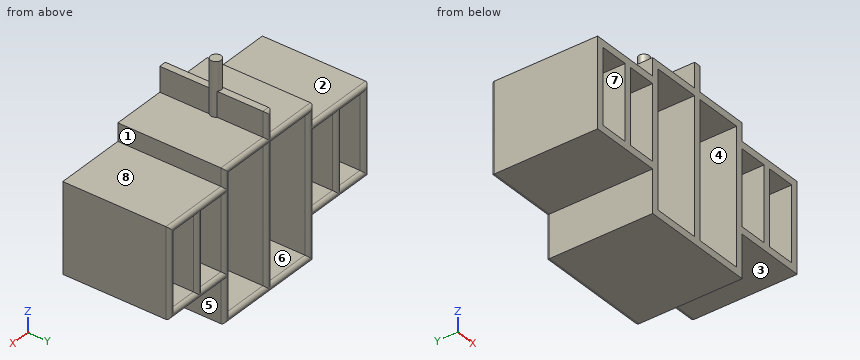
Autodesk Inventor part; units mm, degrees
ref_plane "YZ Plane" through (0, 0, 0) normal (1, 0, 0) x (0, 1, 0)
ref_plane "XZ Plane" through (0, 0, 0) normal (0, 1, 0) x (-1, 0, 0)
ref_plane "XY Plane" through (0, 0, 0) normal (0, 0, 1) x (1, 0, 0)
sketch "Szkic1" plane through (0, 0, 0) normal (0, 1, 0) x (-1, 0, 0)
  line L0 (16.25, 0) -> (-16.25, 0)
  line L1 (-16.25, 0) -> (-16.25, 2)
  line L2 (-16.25, 2) -> (16.25, 2)
  line L3 (16.25, 2) -> (16.25, 0)
  line L4 (-1, 2) -> (1, 2)
  line L5 (1, 2) -> (1, 49)
  line L6 (1, 49) -> (-1, 49)
  line L7 (-1, 49) -> (-1, 2)
  line L8 (16.25, 2) -> (14.25, 2)
  line L9 (14.25, 2) -> (14.25, 42)
  line L10 (14.25, 42) -> (16.25, 42)
  line L11 (16.25, 42) -> (16.25, 2)
  line L12 (-16.25, 2) -> (-14.25, 2)
  line L13 (-14.25, 2) -> (-14.25, 42)
  line L14 (-14.25, 42) -> (-16.25, 42)
  line L15 (-16.25, 42) -> (-16.25, 2)
  line L16 (14.25, 42) -> (1, 42)
  line L17 (1, 42) -> (1, 40)
  line L18 (1, 40) -> (14.25, 40)
  line L19 (14.25, 40) -> (14.25, 42)
  line L20 (-14.25, 42) -> (-1, 42)
  line L21 (-1, 42) -> (-1, 40)
  line L22 (-1, 40) -> (-14.25, 40)
  line L23 (-14.25, 40) -> (-14.25, 42)
  line L24 (16.25, 37) -> (36.25, 37)
  line L25 (36.25, 37) -> (36.25, 12)
  line L26 (36.25, 12) -> (16.25, 12)
  line L27 (16.25, 12) -> (16.25, 37)
  line L28 (-16.25, 37) -> (-36.25, 37)
  line L29 (-36.25, 37) -> (-36.25, 12)
  line L30 (-36.25, 12) -> (-16.25, 12)
  line L31 (-16.25, 12) -> (-16.25, 37)
  circle A0 centre (0, -31.074) radius 80.074
  line L32 (36.25, 37) -> (34.25, 37)
  line L33 (34.25, 37) -> (34.25, 12)
  line L34 (34.25, 12) -> (36.25, 12)
  line L35 (36.25, 12) -> (36.25, 37)
  line L36 (34.25, 37) -> (16.25, 37)
  line L37 (16.25, 37) -> (16.25, 35)
  line L38 (16.25, 35) -> (34.25, 35)
  line L39 (34.25, 35) -> (34.25, 37)
  line L40 (34.25, 12) -> (16.25, 12)
  line L41 (16.25, 12) -> (16.25, 14)
  line L42 (16.25, 14) -> (34.25, 14)
  line L43 (34.25, 14) -> (34.25, 12)
  line L44 (-16.25, 37) -> (-36.25, 37)
  line L45 (-36.25, 37) -> (-36.25, 35)
  line L46 (-36.25, 35) -> (-16.25, 35)
  line L47 (-16.25, 35) -> (-16.25, 37)
  line L48 (-16.25, 12) -> (-36.25, 12)
  line L49 (-36.25, 12) -> (-36.25, 14)
  line L50 (-36.25, 14) -> (-16.25, 14)
  line L51 (-16.25, 14) -> (-16.25, 12)
  line L52 (-36.25, 35) -> (-34.25, 35)
  line L53 (-34.25, 35) -> (-34.25, 14)
  line L54 (-34.25, 14) -> (-36.25, 14)
  line L55 (-36.25, 14) -> (-36.25, 35)
  line L56 (26.25, 35) -> (24.25, 35)
  line L57 (24.25, 35) -> (24.25, 14)
  line L58 (24.25, 14) -> (26.25, 14)
  line L59 (26.25, 14) -> (26.25, 35)
  line L60 (-24.25, 35) -> (-26.25, 35)
  line L61 (-26.25, 35) -> (-26.25, 14)
  line L62 (-26.25, 14) -> (-24.25, 14)
  line L63 (-24.25, 14) -> (-24.25, 35)
  point P0 (0, 0)
  point P1 (0, 0)
  point P2 (0, 2)
  point P3 (7.625, 40)
  point P4 (7.625, 42)
  point P5 (0, 49)
  point P6 (26.25, 37)
  point P7 (26.25, 14)
  point P8 (1, 42)
  point P9 (1, 48.9938)
  point P10 (-1, 48.9938)
  point P11 (-1, 42)
  point P12 (-16.25, 12)
  point P13 (16.25, 12)
  point P14 (-16.25, 14)
  point P15 (16.25, 14)
  dimension "d0" = 32.5
  dimension "d1" = 2
  dimension "d2" = 2
  dimension "d3" = 49
  dimension "d4" = 40
  dimension "d5" = 2
  dimension "d6" = 2
  dimension "d7" = 2
  dimension "d8" = 20
  dimension "d9" = 20
  dimension "d10" = 25
  dimension "d11" = 25
  dimension "d12" = 160.148
  dimension "d13" = 80.074
  dimension "d14" = 5
  dimension "d15" = 5
  dimension "d16" = 2
  dimension "d17" = 2
  dimension "d18" = 2
  dimension "d19" = 2
  dimension "d20" = 2
  dimension "d21" = 2
  dimension "d22" = 2
  dimension "d23" = 8
  dimension "d24" = 8
extrude "Wyciągnięcie proste1" add sketch "Szkic1" along normal blind 30 contours L0 L1 L2 L3 | L2 L9 L10 L11 | L15 L14 L13 L2 | L11 L42 L33 L26 | L30 L29 L50 L15 | L2 L7 A0 L5 | L18 L5 L16 L9 | L33 L24 L25 L26 | L13 L20 L7 L22 | L11 L24 L33 L38 | L57 L38 L59 L42 | L46 L29 L28 L15 | L50 L61 L46 L63 | L29 L46 L53 L50
sketch "Szkic2" plane through (1, 0, 42) normal (0, 0, 1) x (1, 0, 0)
  circle A0 centre (-1, 15) radius 1.5
  line L0 (0, 30) -> (15.25, 30)
  line L1 (0, 0) -> (0, 30)
  point P0 (-1, 0)
  dimension "d27" = 3
  dimension "d30" = 15
  dimension "d31" = 1
extrude "Wyciągnięcie proste2" add sketch "Szkic2" along normal blind 15
fillet "Zaokrąglenie1" radius 1 40 edges at (36.25, 30, 24.5) (34.25, 30, 24.5) (26.25, 30, 37) (30.25, 30, 35) (26.25, 30, 24.5) (20.25, 30, 35) (24.25, 30, 24.5) (30.25, 30, 14) (26.25, 30, 12) (20.25, 30, 14) (1, 30, 45.4969) (0, 30, 49) (-1, 30, 45.4969) (8.625, 30, 42) (16.25, 30, 39.5) (16.25, 30, 24.5) (14.25, 30, 21) (16.25, 30, 6) (7.625, 30, 2) (0, 30, 0) (1, 30, 21) (-1, 30, 21) (7.625, 30, 40) (-7.625, 30, 40) (-8.625, 30, 42) (-16.25, 30, 39.5) (-14.25, 30, 21) (-16.25, 30, 24.5) (-26.25, 30, 37) (-20.25, 30, 35) (-24.25, 30, 24.5) (-26.25, 30, 24.5) (-30.25, 30, 35) (-34.25, 30, 24.5) (-36.25, 30, 24.5) (-30.25, 30, 14) (-26.25, 30, 12) (-20.25, 30, 14) (-16.25, 30, 6) (-7.625, 30, 2)
equation "\"d5\" = d2"
equation "\"d6\" = d2"
equation "\"d9\" = d8"
equation "\"d11\" = d10"
equation "\"d15\" = d14"
equation "\"d16\" = d6"
equation "\"d19\" = d18"
equation "\"d22\" = d21"
properties part number "klapy"
Work out the finished part from the listing and answer in its coordinate system (mm). Face numbers are marked on the shaded views. A direction names the side the tool comes from. Coordinates: 2 decimals unless noted, no trailing zeros.
1) Consider probe 1 along X at (y, z) = (10, 9); probe 2 along Z at (x, y) = (-9.5, 16); probe 3 along X at (y, z) = (15, 36.5). Determine where each line is inside the solid, lowest interval first.
Results:
probe 1: x = -16.25 to -14.25, -1 to 1, 14.25 to 16.25
probe 2: z = 0 to 2, 40 to 42
probe 3: x = -36.25 to -14.25, -1 to 1, 14.25 to 36.25
2) For a pull along Z with two mould halves and no side action, classify the marked faces 5, 6, 7 and 8 as +Z half, -Z half, draft (parallel to the pull), parting line (faces both ways), or undercut.
Results:
face 5: draft
face 6: undercut
face 7: undercut
face 8: +Z half
3) For the marked faces 1, 2, 3 and 4, determine the directions among +Z, -Z, +X, -X, +Y, -Y from which every point of the face is accessible in a straight line to the end or side of a thin tool.
Results:
face 1: +Z, +X, +Y, -Y
face 2: +Z, -X, +Y, -Y
face 3: -Z, +X, +Y, -Y
face 4: +Y, -Y
4) Section B-B (z = 15.5) is taken. Give the number of separate pieces and of enclosed holes in the cut face, plus the area to 3 significant figures.
Results:
separate pieces: 7
enclosed holes: 0
area: 417 mm2
5) Flat-ended cylindrical pins translate along their axes: pin 1 (4.5 mm diameter, centred on x = -8, y = 13, fed in from +Z); pin 2 (2.5 mm diameter, centred on x = -31, y = 15.5, fed in from +Z); pin 3 (6.5 mm diameter, centred on x = -21, y = 16, fed in from -Z). Find the tip coordinate at first contact, or state that the pin passes through.
Results:
pin 1: stops at z = 42
pin 2: stops at z = 37
pin 3: stops at z = 12
